```python
from build123d import *

# Parameters (mm, degrees)
BOSS_EXTRUDE1_START = -1.5
BOSS_EXTRUDE1_DEPTH = 17
CHAMFER1_SIZE       = 0.5
CHAMFER2_SIZE       = 0.5
SKETCH3_R           = 2.25
SKETCH3_R_2         = 3.5
CUT_EXTRUDE1_DEPTH  = 0.25
SKETCH4_R           = 1.5
SKETCH4_R_2         = 2.75
CUT_EXTRUDE2_DEPTH  = 10


with BuildPart() as part:
    # Sketch1 → Boss-Extrude1 (new body)
    with BuildSketch(Plane(origin=(0, 0, 0), x_dir=(1, 0, 0), z_dir=(0, 1, 0)).offset(BOSS_EXTRUDE1_START)):
        Polygon((-119.371877221, -118.892211925), (-105.214028152, -102.711812989), (-112.084182588, -96.700427857), (-126.242031658, -112.880826794), align=None)
    extrude(amount=-BOSS_EXTRUDE1_DEPTH)

    # Chamfer1
    chamfer1_edges = [part.edges().sort_by_distance(p)[0] for p in [
        (-119.371877221, -10, 118.892211925),
        (-105.214028152, -10, 102.711812989),
        (-112.084182588, -10, 96.700427857),
        (-126.242031658, -10, 112.880826794),
    ]]
    chamfer(chamfer1_edges, length=CHAMFER1_SIZE)

    # Chamfer2
    # the kernel refuses this chamfer: 0.5 mm, written as the material it takes off along each edge
    with BuildSketch(Plane(origin=(-104.622622158, -18.5, 103.229293234), x_dir=(-0.6582556384124536, -0.027495876610589123, 0.7522921581856536), z_dir=(-0.7525766947068745, 0, -0.6585046078685219)), Plane(origin=(-126.833437652, -18.5, 112.363346549), x_dir=(0.6582556384124544, -0.027495876610588624, -0.752292158185653), z_dir=(0.7525766947068739, 0, 0.6585046078685227))) as chamfer2_piece_1:
        Polygon((CHAMFER2_SIZE * 0.999621916911, CHAMFER2_SIZE * 0.0274958766106), (-CHAMFER2_SIZE * 0.0274958766106, CHAMFER2_SIZE * 0.999621916911), (0, 0), align=None)
    extrude(amount=10.700525914, mode=Mode.SUBTRACT)
    with BuildSketch(Plane(origin=(-111.566702344, -18.5, 96.109021863), x_dir=(0.7522921581856542, -0.027495876610589123, 0.6582556384124529), z_dir=(-0.6585046078685213, 0, 0.7525766947068752)), Plane(origin=(-119.889357466, -1.5, 119.483617919), x_dir=(0.02069275593768218, -0.9996219169112961, 0.018106161445472113), z_dir=(0.6585046078685223, 0, -0.7525766947068742))) as chamfer2_piece_2:
        Polygon((CHAMFER2_SIZE * 0.999621916911, CHAMFER2_SIZE * 0.0274958766106), (-CHAMFER2_SIZE * 0.0274958766106, CHAMFER2_SIZE * 0.999621916911), (0, 0), align=None)
    extrude(amount=23.071682988, mode=Mode.SUBTRACT)
    with BuildSketch(Plane(origin=(-119.889357466, -18.5, 119.483617919), x_dir=(0.020692755937682127, 0.9996219169112961, 0.018106161445472065), z_dir=(0.6585046078685223, 0, -0.7525766947068742)), Plane(origin=(-111.566702344, -1.5, 96.109021863), x_dir=(0.7522921581856542, 0.027495876610586535, 0.6582556384124529), z_dir=(-0.6585046078685213, 0, 0.7525766947068752))) as chamfer2_piece_3:
        Polygon((CHAMFER2_SIZE * 0.999621916911, -CHAMFER2_SIZE * 0.0274958766106), (-CHAMFER2_SIZE * 0.0274958766106, -CHAMFER2_SIZE * 0.999621916911), (0, 0), align=None)
    extrude(amount=23.071682988, mode=Mode.SUBTRACT)
    with BuildSketch(Plane(origin=(-104.622622158, -1.5, 103.229293234), x_dir=(-0.6582556384124536, 0.027495876610586965, 0.7522921581856536), z_dir=(-0.7525766947068745, 0, -0.6585046078685219)), Plane(origin=(-126.833437652, -1.5, 112.363346549), x_dir=(0.6582556384124544, 0.027495876610586036, -0.752292158185653), z_dir=(0.7525766947068739, 0, 0.6585046078685227))) as chamfer2_piece_4:
        Polygon((CHAMFER2_SIZE * 0.999621916911, -CHAMFER2_SIZE * 0.0274958766106), (-CHAMFER2_SIZE * 0.0274958766106, -CHAMFER2_SIZE * 0.999621916911), (0, 0), align=None)
    extrude(amount=10.700525914, mode=Mode.SUBTRACT)

    # Sketch3 → Cut-Extrude1 (cut)
    with BuildSketch(Plane(origin=(0, -1.5, 0), x_dir=(1, 0, 0), z_dir=(0, 1, 0))):
        with Locations(Location((-110.789245346, -102.151994681, 0), (0, 0, 270))):
            Circle(SKETCH3_R)
        with Locations(Location((-115.728029905, -107.796319891, 0), (0, 0, 270))):
            Circle(SKETCH3_R_2)
        with Locations(Location((-120.666814464, -113.440645102, 0), (0, 0, 270))):
            Circle(SKETCH3_R)
    extrude(amount=-CUT_EXTRUDE1_DEPTH, mode=Mode.SUBTRACT)

    # Sketch4 → Cut-Extrude2 (cut)
    with BuildSketch(Plane(origin=(0, -1.5, 0), x_dir=(1, 0, 0), z_dir=(0, 1, 0))):
        with Locations(Location((-110.789245346, -102.151994681, 0), (0, 0, 270))):
            Circle(SKETCH4_R)
        with Locations(Location((-115.728029905, -107.796319891, 0), (0, 0, 270))):
            Circle(SKETCH4_R_2)
        with Locations(Location((-120.666814464, -113.440645102, 0), (0, 0, 270))):
            Circle(SKETCH4_R)
    extrude(amount=-CUT_EXTRUDE2_DEPTH, mode=Mode.SUBTRACT)


solid = part.part
```
Input: part model. Units: mm. Frame: model coordinates. A direction names the side the tool comes from. Round coordinates to 2 decimals unless told otherwise and drop trailing zeros. Write each loop counter-clockwise with the first axis right and the second up, starting at its lowest first coordinate (ties: lowest second). Pieces come first, ordered by that corner, then holes. Notation, with made-up numbers: M 10.25,-6 L 43.25,-6 A34 ccw 43.25,27 Z; hole C -34,28 d8. An arc over 180 degrees is marked long. Write each question's results on one line, items separated by ' | '.
Q1. Draft query along X for faces 3 (the face through (-112.58, -1.75, 110.75)), 4 (the face through (-116, -18.5, 108)), 5 (the face through (-121, -11.5, 113)), 6 (the face through (-122.85, -9.89, 115.85)). Return one class per face: released by +X, released by -X, zero draft, split by the parting line, or undercut.
Results:
face 3: released by +X | face 4: zero draft | face 5: undercut | face 6: released by -X
Q2. Access query for faces 1 (the face through (-111, -1.75, 104)), 2 (the face through (-118.88, -1.75, 104.85)). Directions: +Z, -Z, +X, -X, +Y, -Y. A direction counts if a zero-diameter tool reaches every point of the face in a straight line with its end or side. Return the directions, or none.
Results:
face 1: +Y | face 2: -Z, -X, +Y
Q3. Section query C-C (x = -117.5). Return loops of the section in (y, z), and give its area (3 significant figures).
Results:
outline: M -18.5,103.65 L -18,102.89 L -2,102.89 L -1.5,103.65 L -1.5,104.78 L -1.75,104.78 L -1.75,105.69 L -11.5,105.69 L -11.5,109.9 L -1.75,109.9 L -1.75,110.81 L -1.5,110.81 L -1.5,115.99 L -2,116.75 L -18,116.75 L -18.5,115.99 Z | area: 192 mm^2
Q4. Line query: line 1 along Z through (x, y) = (-113.75, -11.25); line 2 along Z through (x, y) = (-119.5, -6.75); line 3 along X through (y, z) = (-3.25, 107). Output: solid intervals per line, ascending.
Results:
line 1: z = 98.6 to 105.89, 109.71 to 112.47 | line 2: z = 105.18 to 112.5, 114.38 to 118.55 | line 3: x = -121.1 to -118.36, -113.1 to -108.97
Q5. Section query B-B (z = 108.25). Return loops of the section in (x, y).
Results:
outline: M -122.19,-18 L -121.53,-18.5 L -110.72,-18.5 L -110.06,-18 L -110.06,-2 L -110.72,-1.5 L -112.26,-1.5 L -112.26,-1.75 L -113.02,-1.75 L -113.02,-11.5 L -118.44,-11.5 L -118.44,-1.75 L -119.2,-1.75 L -119.2,-1.5 L -121.53,-1.5 L -122.19,-2 Z
Q6. Section query A-A (y = -14). Return loops of the section in (x, z), and give its area (3 significant figures).
Results:
outline: M -125.91,112.5 L -112.41,97.08 L -111.71,97.03 L -105.59,102.38 L -105.54,103.09 L -119.04,118.52 L -119.75,118.56 L -125.87,113.21 Z | area: 196 mm^2
Q7. Section query D-D (y = -6.75). Return loops of the section in (x, z).
Results:
outline: M -125.91,112.5 L -112.41,97.08 L -111.71,97.03 L -105.59,102.38 L -105.54,103.09 L -119.04,118.52 L -119.75,118.56 L -125.87,113.21 Z; hole C -120.67,113.44 d3; hole C -115.73,107.8 d5.5; hole C -110.79,102.15 d3
Q8. Pin query (flat end, axial travel): P1, Ø1.3, axis at x = -121, z = 114, coming from the +Y side; P2, Ø3, axis at x = -122, y = -4.5, coming from the -Z side; P3, Ø3, axis at x = -114.5, z = 109, coming from the +Y side. Return the tip coordinate at first contact, or that it passes through.
Results:
P1: stops at y = -11.5 | P2: stops at z = 106.32 | P3: stops at y = -1.75
